Can you work these out from the model? Positions are in its coordinate system, mm. A direction names the side the tool comes from. Round coordinates to 2 decimals unless told otherwise and drop trailing zeros. Loops run counter-clockwise (first coordinate to the right, second up) from the corner with the lowest first, then second, coordinate; pieces in that order, holes last. Notation, with made-up numbers: M -22,5 L 7,5 A14 ccw 7,11 Z; hole C 26.25,23.25 d7. An arc over 180 degrees is marked long. Return JSON: item names as keys, results as strings.
```python
from build123d import *

# Parameters (mm, degrees)
F1_DEPTH = 25
F3_R     = 2.5
F4_DEPTH = 25
F2_R     = 2.5
F5_DEPTH = 25


# Not quite as in the source:
# - ends of sketch curves that miss each other by under 0.0002 mm in the source are joined


with BuildPart() as f1:
    # F0 (on Front) → F1 (new body)
    with BuildSketch(Plane.XZ):
        with BuildLine():
            Line((40, 55), (55, 55))
            Line((55, 55), (55, 62.0000141774))
            Line((55, 62.0000141774), (-55, 62.0000141774))
            ThreePointArc((-55, 62.0000141774), (-59.9497599972, 59.9497599972), (-62.0000177185, 55))
            Line((-62.0000177185, 55), (-62.0000141774, -55))
            ThreePointArc((-62.0000141774, -55), (-59.9497574932, -59.9497574932), (-55, -62.0000141774))
            Line((-55, -62.0000141774), (-55, -55))
            Line((-55, -55), (-55, -40))
            Line((-55, -40), (-55, -35))
            Line((-55, -35), (-55, 35))
            Line((-55, 35), (-55, 40))
            Line((-55, 40), (-55, 55))
            Line((-55, 55), (-40, 55))
            Line((-40, 55), (-35, 55))
            Line((-35, 55), (35, 55))
            Line((35, 55), (40, 55))
        make_face()
        with BuildLine():
            Line((55, 62.0000141774), (55, 55))
            Line((55, 55), (55, 40))
            Line((55, 40), (55, 35))
            Line((55, 35), (55, -35))
            Line((55, -35), (55, -40))
            Line((55, -40), (55, -55))
            Line((55, -55), (40, -55))
            Line((40, -55), (35, -55))
            Line((35, -55), (-35, -55))
            Line((-35, -55), (-40, -55))
            Line((-40, -55), (-55, -55))
            Line((-55, -55), (-55, -62.0000141774))
            Line((-55, -62.0000141774), (55, -62.0000141774))
            ThreePointArc((55, -62.0000141774), (59.9497599972, -59.9497599972), (62.0000177185, -55))
            Line((62.0000177185, -55), (62.0000141774, 55))
            ThreePointArc((62.0000141774, 55), (59.9497574932, 59.9497574932), (55, 62.0000141774))
        make_face()
        Polygon((-55, 35), (-35, 55), (-40, 55), (-55, 40), align=None)
        Polygon((55, 40), (40, 55), (35, 55), (55, 35), align=None)
        Polygon((55, -40), (55, -35), (35, -55), (40, -55), align=None)
        Polygon((-35, -55), (-55, -35), (-55, -40), (-40, -55), align=None)
    extrude(amount=F1_DEPTH)

    # F3 (on face) → F4 (cut)
    with BuildSketch(Plane(origin=(0, 0, -62.0000141774), x_dir=(1, 0, 0), z_dir=(0, 0, -1))):
        with Locations((-7.5450468063, 12.5)):
            Circle(F3_R)
    extrude(amount=-F4_DEPTH, mode=Mode.SUBTRACT)

    # F2 (on face) → F5 (cut)
    with BuildSketch(Plane.XY.offset(62.0000141774)):
        with Locations((0, -12.5)):
            Circle(F2_R)
    extrude(amount=-F5_DEPTH, mode=Mode.SUBTRACT)


solid = f1.part
```
Q1. Suppose I cut it at A-A, the plane x = 0. Please give me the cut outline in (y, z).
Results:
{"outline": "M -25,-62 L 0,-62 L 0,-55 L -25,-55 Z; M -25,55 L -15,55 L -15,62 L -25,62 Z; M -10,55 L 0,55 L 0,62 L -10,62 Z"}
Q2. Thinking about a two-plate mould opening in X: for faces 1 (the cylindrical face through (-8.09, -10.06, -58.55)), 2 (the flat face through (1, -10, 62)), 3 (the cylindrical face through (-60, -12.3, -59.9)), which applies, pulls with the +X half, pulls with the -X half, needs draft (parallel to the pull), parting line crosses it, or undercut?
Results:
{"face 1": "undercut", "face 2": "needs draft", "face 3": "pulls with the -X half"}
Q3. If I drill on line 1 along Z through (x, y) = (12, -12.25); line 2 along Y through (x, z) = (0, 60), over which ranges is the centre line in solid material (lowest first)?
Results:
{"line 1": "z = -62 to -55, 55 to 62", "line 2": "y = -25 to -15, -10 to 0"}
Q4. On a 3-axis mill with a long thin cutter (end or side, diameter ignored), from which of +Z, -Z, +X, -X, +Y, -Y can I reach the whole of each face in a straight line? I mean faces 4 (the flat face through (-1, -12, -62)), 5 (the flat face through (-0.5, -9.5, 55)). Say none if no direction works.
Results:
{"face 4": "-Z, +X, -X, +Y, -Y", "face 5": "+Y, -Y"}
Q5. I'm going to push a flat-ended pin straight in: pin 1 Ø4 at (x, y) = (0, -12.5) entering from +Z. Where does the tip first touch, or does it pass through?
Results:
{"pin 1": "stops at z = -55"}
Q6. Suppose I cut it at B-B, the plane z = 51. Please give me the cut outline in (x, y), plus the area to 3 significant figures.
Results:
{"outline": "M -62,-25 L -55,-25 L -55,0 L -62,0 Z; M -44,-25 L -39,-25 L -39,0 L -44,0 Z; M 39,-25 L 44,-25 L 44,0 L 39,0 Z; M 55,-25 L 62,-25 L 62,0 L 55,0 Z", "area": "600 mm2"}
Q7. Suppose I cut it at D-D, the plane z = -13. Please give me the cut outline in (x, y).
Results:
{"outline": "M -62,-25 L -55,-25 L -55,0 L -62,0 Z; M 55,-25 L 62,-25 L 62,0 L 55,0 Z"}
Q8. Suppose I cut it at C-C, the plane y = -19. Please give me the cut outline in (x, z).
Results:
{"outline": "M -62,-55 A7 ccw -55,-62 L 55,-62 A7 ccw 62,-55 L 62,55 A7 ccw 55,62 L -55,62 A7 ccw -62,55 Z; hole M -55,-55 L -40,-55 L -55,-40 Z; hole M -55,-35 L -35,-55 L 35,-55 L 55,-35 L 55,35 L 35,55 L -35,55 L -55,35 Z; hole M -55,40 L -40,55 L -55,55 Z; hole M 40,-55 L 55,-55 L 55,-40 Z; hole M 40,55 L 55,40 L 55,55 Z"}
